```python
from build123d import *

# Parameters (mm, degrees)
SKETCH1_W                 = 30
SKETCH1_H                 = 21.65
BOSS_EXTRUDE1_DEPTH       = 90
M4X0_7_TAPPED_HOLE1_D     = 3.3
M4X0_7_TAPPED_HOLE1_DEPTH = 10
M4X0_7_TAPPED_HOLE1_TIP   = 0.991420021
M4X0_7_TAPPED_HOLE2_D     = 3.3
M4X0_7_TAPPED_HOLE2_DEPTH = 12
M4X0_7_TAPPED_HOLE2_TIP   = 0.991420021
SKETCH7_W                 = 20.05
SKETCH7_H                 = 55
CUT_EXTRUDE1_DEPTH        = 96.483928622
CHAMFER1_SIZE             = 5
M4X0_7_TAPPED_HOLE3_D     = 3.3
M4X0_7_TAPPED_HOLE3_DEPTH = 10
M4X0_7_TAPPED_HOLE3_TIP   = 0.991420021
M4X0_7_TAPPED_HOLE4_D     = 3.3
M4X0_7_TAPPED_HOLE4_DEPTH = 8
M4X0_7_TAPPED_HOLE4_TIP   = 0.991420021


with BuildPart() as part:
    # Sketch1 → Boss-Extrude1 (new body)
    with BuildSketch(Plane(origin=(0, 0, 0), x_dir=(1, 0, 0), z_dir=(0, 1, 0))):
        Rectangle(SKETCH1_W, SKETCH1_H)
    extrude(amount=BOSS_EXTRUDE1_DEPTH)

    # M4x0.7 Tapped Hole1
    with Locations(Plane(origin=(0, 90, 0), x_dir=(1, 0, 0), z_dir=(0, 1, 0))):
        with Locations((-10, 5.825), (10, 5.825)):
            Hole(M4X0_7_TAPPED_HOLE1_D / 2, depth=M4X0_7_TAPPED_HOLE1_DEPTH)
            with Locations((0, 0, -(M4X0_7_TAPPED_HOLE1_DEPTH + M4X0_7_TAPPED_HOLE1_TIP / 2))):  # 118° drill point
                Cone(0, M4X0_7_TAPPED_HOLE1_D / 2, M4X0_7_TAPPED_HOLE1_TIP, mode=Mode.SUBTRACT)

    # M4x0.7 Tapped Hole2
    with Locations(Plane(origin=(0, 0, 0), x_dir=(-1, 0, 0), z_dir=(0, -1, 0))):
        with Locations((-10, -0.825), (10, -0.825)):
            Hole(M4X0_7_TAPPED_HOLE2_D / 2, depth=M4X0_7_TAPPED_HOLE2_DEPTH)
            with Locations((0, 0, -(M4X0_7_TAPPED_HOLE2_DEPTH + M4X0_7_TAPPED_HOLE2_TIP / 2))):  # 118° drill point
                Cone(0, M4X0_7_TAPPED_HOLE2_D / 2, M4X0_7_TAPPED_HOLE2_TIP, mode=Mode.SUBTRACT)

    # Sketch7 → Cut-Extrude1 (cut, through all)
    with BuildSketch(Plane(origin=(15, 0, 0), x_dir=(0, 0, -1), z_dir=(1, 0, 0))):
        with Locations((0, 45)):
            Rectangle(SKETCH7_W, SKETCH7_H)
    extrude(amount=-CUT_EXTRUDE1_DEPTH, mode=Mode.SUBTRACT)

    # Chamfer1
    chamfer1_edges = [part.edges().sort_by_distance(p)[0] for p in [
        (0, 72.5, -10.025),
        (0, 17.5, -10.025),
        (0, 17.5, 10.025),
        (0, 72.5, 10.025),
    ]]
    chamfer(chamfer1_edges, length=CHAMFER1_SIZE)

    # M4x0.7 Tapped Hole3
    with Locations(Plane.XY.offset(10.825)):
        with Locations((-10, 15), (10, 15), (10, 75), (-10, 75)):
            Hole(M4X0_7_TAPPED_HOLE3_D / 2, depth=M4X0_7_TAPPED_HOLE3_DEPTH)
            with Locations((0, 0, -(M4X0_7_TAPPED_HOLE3_DEPTH + M4X0_7_TAPPED_HOLE3_TIP / 2))):  # 118° drill point
                Cone(0, M4X0_7_TAPPED_HOLE3_D / 2, M4X0_7_TAPPED_HOLE3_TIP, mode=Mode.SUBTRACT)

    # M4x0.7 Tapped Hole4
    with Locations(Plane(origin=(15, 0, 0), x_dir=(0, 0, -1), z_dir=(1, 0, 0))):
        with Locations((5.825, 12.5), (5.825, 77.5)):
            Hole(M4X0_7_TAPPED_HOLE4_D / 2, depth=M4X0_7_TAPPED_HOLE4_DEPTH)
            with Locations((0, 0, -(M4X0_7_TAPPED_HOLE4_DEPTH + M4X0_7_TAPPED_HOLE4_TIP / 2))):  # 118° drill point
                Cone(0, M4X0_7_TAPPED_HOLE4_D / 2, M4X0_7_TAPPED_HOLE4_TIP, mode=Mode.SUBTRACT)


solid = part.part
```
Source: CAD feature listing. Evaluate the final solid. Frame: model axes, mm. A direction names the side the tool comes from. Round coordinates to 2 decimals unless told otherwise and drop trailing zeros. Write each loop counter-clockwise with the first axis right and the second up, starting at its lowest first coordinate (ties: lowest second). Pieces come first, ordered by that corner, then holes. Notation, with made-up numbers: M 16.5,22.5 L 38.5,22.5 A16 ccw 38.5,37.5 Z; hole C -11,34.5 d9. An arc over 180 degrees is marked long. Use CSV: the item, a comma, the result in double quotes. Start each with the question number.
Q1. First-contact query: P1, Ø4, axis at y = 12.5, z = -5.825, coming from the +X side; P2, Ø2.5, axis at x = -10, z = -5.825, coming from the +Y side. Flat tips, straight axial feed; report the tip coordinate or a pass-through.
Q2. Cut plane B-B on x = -4. Output: boundary loops of the cut face in (y, z) (3 decimals).
Q3. Cut plane A-A on y = 47. Output: boundary loops of the cut face in (x, z) (3 decimals), plus the area to 3 significant figures.
Q4. Access query for faces 1 (the face through (-8.476, 6.084, 1.457)), 2 (the face through (0.21, 69.965, 7.56)), 3 (the face through (-9.785, 76.636, 5.755)). Directions: +Z, -Z, +X, -X, +Y, -Y. A direction counts if a zero-diameter tool reaches every point of the face in a straight line with its end or side. Return the directions, or none.
Q5. Pull-direction query (Z, two-part tool) for faces 4 (the face through (-9.727, 75.086, 0.006)), 5 (the face through (-10.265, 12.819, 0.935)), 6 (the face through (0, 0, 0)); classes: +Z half, -Z half, draft (parallel to the pull), parting line (faces both ways), or undercut.
Q6. Cut plane C-C on z = -2. Output: boundary loops of the cut face in (x, y).
Q7. Line query: line 1 (Y direction, x = -10, z = 5); line 2 (Z direction, x = 8.5, y = 42) (3 decimals); line 3 (Y direction, x = 10, z = 6.5) (3 decimals). Output: solid intervals per line, ascending. Write a range as from..to.
Results found:
1,P1,"x = 15"
1,P2,"y = 79.76"
2,outline,"M 0,-10.825 L 90,-10.825 L 90,10.825 L 0,10.825 Z; hole M 17.5,-5.025 L 22.5,-10.025 L 67.5,-10.025 L 72.5,-5.025 L 72.5,5.025 L 67.5,10.025 L 22.5,10.025 L 17.5,5.025 Z"
3,outline,"M -15,-10.825 L 15,-10.825 L 15,-10.025 L -15,-10.025 Z; M -15,10.025 L 15,10.025 L 15,10.825 L -15,10.825 Z"
3,area,"48.0 mm^2"
4,face 1,"-Y"
4,face 2,"+X, -X"
4,face 3,"+Z"
5,face 4,"+Z half"
5,face 5,"undercut"
5,face 6,"draft"
6,outline,"M -15,0 L 15,0 L 15,17.5 L -15,17.5 Z; M -15,72.5 L 15,72.5 L 15,90 L -15,90 Z"
7,line 1,"0..13.35, 16.65..17.5, 72.5..73.35, 76.65..90"
7,line 2,"-10.825..-10.025, 10.025..10.825"
7,line 3,"0..13.35, 16.65..18.975, 71.025..73.35, 76.65..90"
